Autodesk Inventor part; units mm, degrees
ref_plane "YZ Plane" through (0, 0, 0) normal (1, 0, 0) x (0, 1, 0)
ref_plane "XZ Plane" through (0, 0, 0) normal (0, 1, 0) x (-1, 0, 0)
ref_plane "XY Plane" through (0, 0, 0) normal (0, 0, 1) x (1, 0, 0)
sketch "スケッチ1" plane through (0, 0, 0) normal (1, 0, 0) x (0, 1, 0)
  line L0 (0, 0) -> (50, 0)
  line L1 (50, 0) -> (50, 20)
  line L2 (50, 20) -> (0, 20) construction
  line L3 (0, 20) -> (0, 0)
  line L4 (0, 0) -> (20, 0)
  line L5 (20, 0) -> (20, 30) construction
  line L6 (20, 30) -> (0, 30)
  line L7 (0, 30) -> (0, 0)
  line L8 (20, 30) -> (50, 20)
  dimension "d0" = 20
  dimension "d1" = 20
  dimension "d2" = 30
  dimension "d3" = 30
extrude "押し出し1" add sketch "スケッチ1" along normal blind 2
sketch "スケッチ2" plane through (2, 0, 0) normal (1, 0, 0) x (0, 0, -1)
  line L0 (-30, 20) -> (-30, 0)
  line L1 (-30, 10) -> (0, 10) construction
  line L2 (0, 0) -> (0, 50)
  line L3 (0, 50) -> (-20, 50)
  line L4 (-10, 50) -> (-10, 0) construction
  line L5 (-30, 0) -> (0, 0)
  point P0 (-25, 10)
  point P1 (-5, 10)
  point P2 (-10, 25)
  point P3 (-10, 45)
  dimension "d6" = 20
  dimension "d7" = 5
  dimension "d8" = 20
  dimension "d9" = 5
hole "穴1" at (2, 10, 25) at (2, 10, 5) at (2, 25, 10) at (2, 45, 10) direction (-1, 0, 0) diameter 3.2 end through all
properties part number "FrameJoint2020" material "アルミニウム 6061"
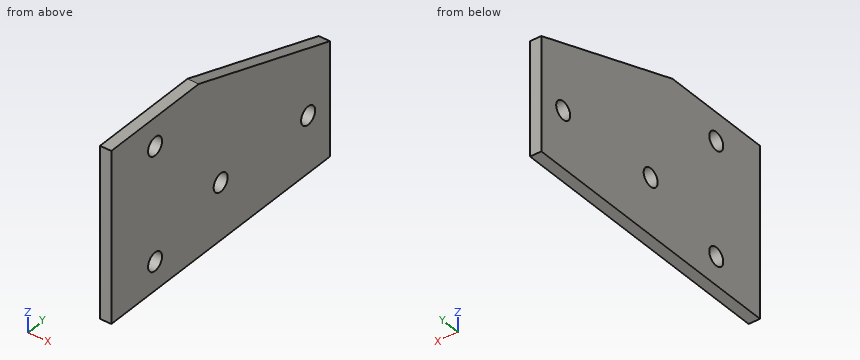
Geometry check sheet. Reference: the model listing, model coordinates, mm. Round coordinates to 2 decimals unless told otherwise and drop trailing zeros. Write each loop counter-clockwise with the first axis right and the second up, starting at its lowest first coordinate (ties: lowest second). Pieces come first, ordered by that corner, then holes. Notation, with made-up numbers: (2.25, -40) - (45.25, -40) arc R21 ccw to (45.25, -14) - close; hole circle Ø7 at (-13, 28.5). An arc over 180 degrees is marked (long way). One line per item, written item: value.
1. Cross-section at C-C on x = 0.65. Record the boundary of the cut face in (y, z).
The answers:
outline: (0, 0) - (50, 0) - (50, 20) - (20, 30) - (0, 30) - close; hole circle Ø3.2 at (10, 5); hole circle Ø3.2 at (10, 25); hole circle Ø3.2 at (25, 10); hole circle Ø3.2 at (45, 10)
2. Cross-section at A-A on y = 10. Record the boundary of the cut face in (x, z).
The answers:
outline: (0, 0) - (2, 0) - (2, 3.4) - (0, 3.4) - close; (0, 6.6) - (2, 6.6) - (2, 23.4) - (0, 23.4) - close; (0, 26.6) - (2, 26.6) - (2, 30) - (0, 30) - close
3. Cross-section at D-D on z = 10. Record the boundary of the cut face in (x, y).
The answers:
outline: (0, 0) - (2, 0) - (2, 23.4) - (0, 23.4) - close; (0, 26.6) - (2, 26.6) - (2, 43.4) - (0, 43.4) - close; (0, 46.6) - (2, 46.6) - (2, 50) - (0, 50) - close
4. Depth check by flat-ended pin: pin 1 Ø1.5 at (y, z) = (40.5, 25) entering from +X. Enter the tip coordinate at first touch or a pass-through.
The answers:
pin 1: passes through
5. Cross-section at B-B on z = 25. Record the boundary of the cut face in (x, y), and give its area (3 significant figures).
The answers:
outline: (0, 0) - (2, 0) - (2, 8.4) - (0, 8.4) - close; (0, 11.6) - (2, 11.6) - (2, 35) - (0, 35) - close
area: 63.6 mm^2
6. Scan lines: L1, parallel to Y at x = 1.25, z = 10; L2, parallel to Z at x = 1.45, y = 10; L3, parallel to Y at x = 0.65, z = 5. Record each from-to range of solid material in increasing order.
The answers:
L1: y = 0 to 23.4, 26.6 to 43.4, 46.6 to 50
L2: z = 0 to 3.4, 6.6 to 23.4, 26.6 to 30
L3: y = 0 to 8.4, 11.6 to 50
